Verification items for this drawing (mm, ordinates from the low corner). Coordinates: 2 decimals unless noted, no trailing zeros. Loops run counter-clockwise (first coordinate to the right, second up) from the corner with the lowest first, then second, coordinate; pieces in that order, holes last. Notation, with made-up numbers: (48, 36) - (89, 36) arc R24 cw to (89, 70) - close; hole circle Ø10 at (-2, -28). An arc over 180 degrees is marked (long way). Write each question's results on one line, items separated by ' | '. Start each with the question number.
(1) Sectioned sample at C-C (z = 40). Enter the section's corners in (x, y).
(2) Sectioned sample at B-B (y = 1.1). Enter the section's corners in (x, z), plus the area to 3 significant figures.
(3) Sectioned sample at D-D (z = 82). Enter the section's corners in (x, y).
(4) Material ranges on probe 1 along X at (y, z) = (3, 40); probe 2 along X at (y, z) = (1.95, 82); probe 3 along Z at (x, y) = (44.5, 0.65), recorded low to high.
(5) Sectioned sample at A-A (x = 15). Enter the section's corners in (y, z).
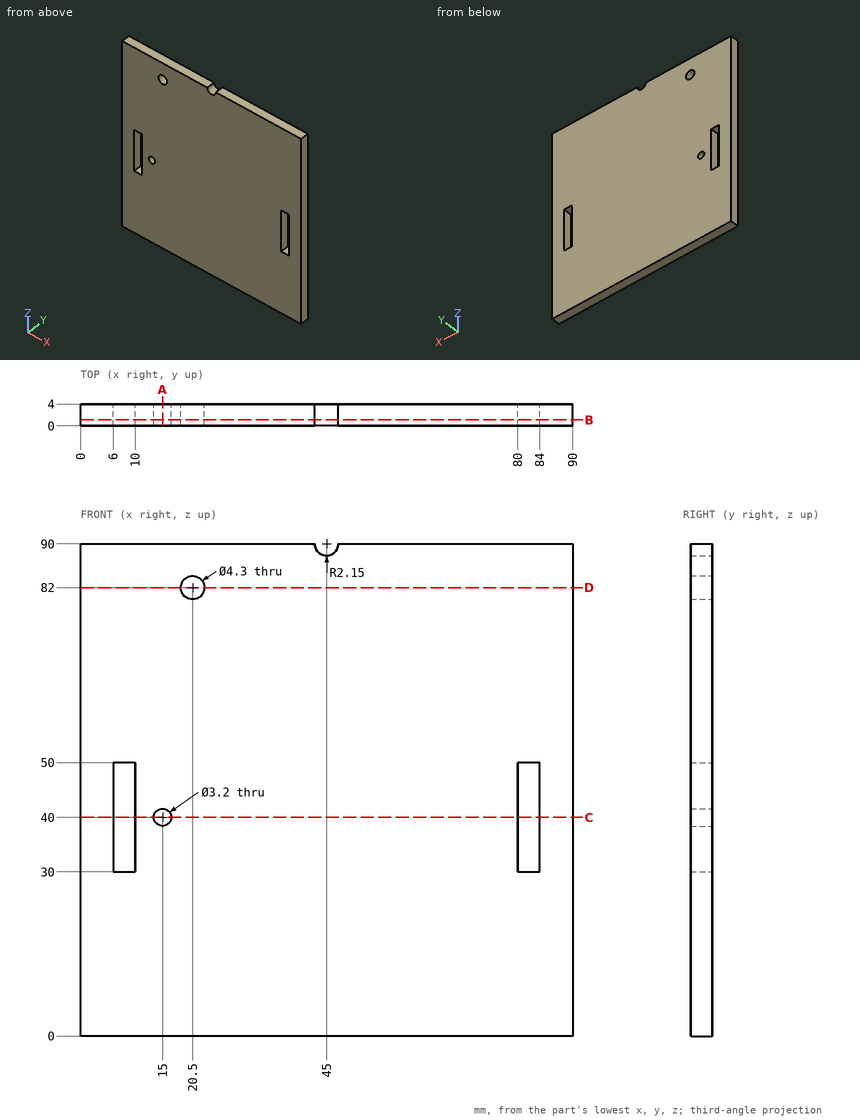
Outcome:
1) outline: (0, 0) - (6, 0) - (6, 4) - (0, 4) - close; (10, 0) - (13.4, 0) - (13.4, 4) - (10, 4) - close; (16.6, 0) - (80, 0) - (80, 4) - (16.6, 4) - close; (84, 0) - (90, 0) - (90, 4) - (84, 4) - close
2) outline: (0, 0) - (90, 0) - (90, 90) - (47.15, 90) arc R2.15 cw to (42.85, 90) - (0, 90) - close; hole (6, 30) - (10, 30) - (10, 50) - (6, 50) - close; hole circle Ø3.2 at (15, 40); hole circle Ø4.3 at (20.5, 82); hole (80, 30) - (84, 30) - (84, 50) - (80, 50) - close | area: 7,910 mm2
3) outline: (0, 0) - (18.35, 0) - (18.35, 4) - (0, 4) - close; (22.65, 0) - (90, 0) - (90, 4) - (22.65, 4) - close
4) probe 1: x = 0 to 6, 10 to 13.4, 16.6 to 80, 84 to 90 | probe 2: x = 0 to 18.35, 22.65 to 90 | probe 3: z = 0 to 87.91
5) outline: (0, 0) - (4, 0) - (4, 38.4) - (0, 38.4) - close; (0, 41.6) - (4, 41.6) - (4, 90) - (0, 90) - close
